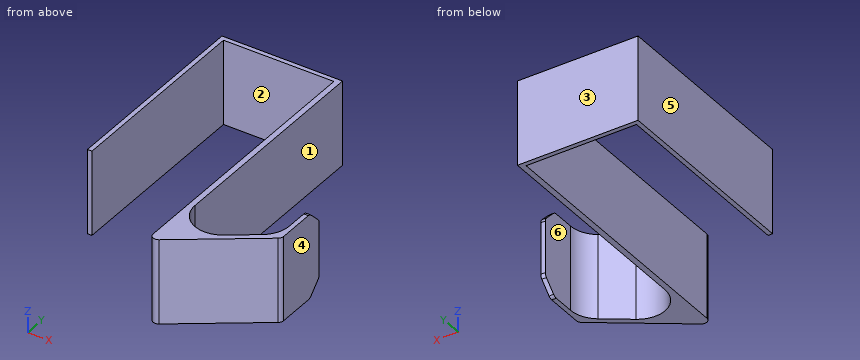
```python
from build123d import *

# Parameters (mm, degrees)
BOSS_EXTRU_1_DEPTH = 30
CONG_1_R           = 10
CHANFREIN1_SIZE    = 5
CONG_2_R           = 2


with BuildPart() as part:
    # Esquisse1 → Boss.-Extru.1 (new body)
    with BuildSketch(Plane.XY):
        Polygon((-19.55, 43.689057372), (-19.55, 113.689057372), (19.55, 113.689057372), (19.55, 13.689057372), (52.316081772, 36.632114826), (52.316081772, 56.632114826), (50.716081772, 56.632114826), (50.716081772, 37.953331942), (21.55, 17.531021626), (21.55, 115.289057372), (-21.15, 115.289057372), (-21.15, 43.689057372), align=None)
    extrude(amount=BOSS_EXTRU_1_DEPTH)

    # Congé1
    cong_1_edges = [part.edges().sort_by_distance(p)[0] for p in [
        (21.55, 17.531021626, 15),
        (50.716081772, 37.953331942, 15),
    ]]
    fillet(cong_1_edges, radius=CONG_1_R)

    # Chanfrein1
    chanfrein1_edges = [part.edges().sort_by_distance(p)[0] for p in [
        (51.516081772, 56.632114826, 0),
        (51.516081772, 56.632114826, 30),
    ]]
    chamfer(chanfrein1_edges, length=CHANFREIN1_SIZE)

    # Congé2
    cong_2_edges = [part.edges().sort_by_distance(p)[0] for p in [
        (52.316081772, 36.632114826, 15),
        (19.55, 13.689057372, 15),
        (51.516081772, 56.632114826, 25),
        (51.516081772, 56.632114826, 5),
        (51.516081772, 51.632114826, 0),
        (51.516081772, 51.632114826, 30),
    ]]
    fillet(cong_2_edges, radius=CONG_2_R)


solid = part.part
```
Could you check a few things on this model? Use its own coordinates, in mm. Face numbers are marked on the shaded views. A direction names the side the tool comes from. Give positions to 0.01 mm unless a question says otherwise; leave off trailing zeros. Loops run counter-clockwise (first coordinate to the right, second up) from the corner with the lowest first, then second, coordinate; pieces in that order, holes last. Notation, with made-up numbers: (69, 67) - (110, 67) arc R9 ccw to (110, 83) - close; hole circle Ø4 at (-8.5, 49.25). An arc over 180 degrees is marked (long way). Use one line per item in the form item = value.
1. I need wall thicknesses on probe 1 along X at (y, z) = (55, 24); probe 2 along X at (y, z) = (107.5, 6.25). Which ranges of each line are inside material? Lowest first, please.
Response values:
probe_1 = -21.15 to -19.55, 19.55 to 21.55, 50.72 to 52.32
probe_2 = -21.15 to -19.55, 19.55 to 21.55
2. On a 3-axis mill with a long thin cutter (end or side, diameter ignored), from which of +Z, -Z, +X, -X, +Y, -Y can I reach the whole of each face in a straight line? I mean the marked faces 1, 2 and 3. Say none if no direction works.
Response values:
face_1 = +Z, -Z, +Y
face_2 = +Z, -Z, -Y
face_3 = +Z, -Z, +X, -X, +Y
3. I want a section at D-D (x = -1.5). Please give me the cut outline in (y, z), and give its area (3 significant figures).
Response values:
outline = (113.69, 0) - (115.29, 0) - (115.29, 30) - (113.69, 30) - close
area = 48.0 mm²
4. I want a section at C-C (z = 21.5). Please give me the cut outline in (x, y), and give its area (3 significant figures).
Response values:
outline = (-21.15, 43.69) - (-19.55, 43.69) - (-19.55, 113.69) - (19.55, 113.69) - (19.55, 17.53) arc R2 ccw to (22.7, 15.89) - (51.46, 36.03) arc R2 ccw to (52.32, 37.67) - (52.32, 56.63) - (50.72, 56.63) - (50.72, 43.16) arc R10 cw to (46.45, 34.97) - (37.29, 28.55) arc R10 cw to (21.55, 36.74) - (21.55, 115.29) - (-21.15, 115.29) - close
area = 567 mm²
5. Thinking about a two-plate mould opening in X: for the marked faces 4, 5 and 6, which applies, released by +X, released by -X, zero draft, split by the parting line, or undercut?
Response values:
face_4 = released by +X
face_5 = released by -X
face_6 = undercut
6. I'm going to push flat-ended pins straight in: pin 1 Ø9 at (x, z) = (0.5, 15) entering from -Y; pin 2 Ø0.8 at (x, z) = (-20, 19.5) entering from -Y; pin 3 Ø1.8 at (x, z) = (51, 12.5) entering from +Y. Where does each tip first touch, or does it pass through?
Response values:
pin_1 = 113.69
pin_2 = 43.69
pin_3 = 56.63
7. I want a section at A-A (y = 71). Please give me the cut outline in (x, z), and give its area (3 significant figures).
Response values:
outline = (-21.15, 0) - (-19.55, 0) - (-19.55, 30) - (-21.15, 30) - close; (19.55, 0) - (21.55, 0) - (21.55, 30) - (19.55, 30) - close
area = 108 mm²
8. I want a section at B-B (y = 49.5). Please give me the cut outline in (x, z), and give its area (3 significant figures).
Response values:
outline = (-21.15, 0) - (-19.55, 0) - (-19.55, 30) - (-21.15, 30) - close; (19.55, 0) - (21.55, 0) - (21.55, 30) - (19.55, 30) - close; (50.72, 0) - (52.32, 0) - (52.32, 30) - (50.72, 30) - close
area = 156 mm²
